Check sheet for the modelled part. Datum: model origin and axes. Units: mm. A direction names the side the tool comes from. Round coordinates to 2 decimals unless told otherwise and drop trailing zeros. Order: outer loops, then holes, each group sorted by start corner. A loop starts at its lowest first (then second) coordinate and runs counter-clockwise, first axis right, second up. Notation, with made-up numbers: (76, 30) -> (100, 30) arc R23 ccw to (100, 49) -> close; hole circle Ø7 at (56.25, -12.5). An arc over 180 degrees is marked (long way). Answer in a Markdown table with one row per item.
from build123d import *

# Parameters (mm, degrees)
BOSS_EXTRUDE1_DEPTH   = 6.35
SKETCH2_W             = 82.55
SKETCH2_H             = 9.525
BOSS_EXTRUDE2_DEPTH   = 50.8
CHAMFER1_SIZE         = 9.525
F_8_CLEARANCE_HOLE1_D = 4.9149
CUT_EXTRUDE1_REACH    = 223.791
SKETCH5_R             = 6.35
F_8_CLEARANCE_HOLE2_D = 4.9149
CHAMFER2_SIZE         = 2.54


with BuildPart() as part:
    # Sketch1 → Boss-Extrude1 (new body)
    with BuildSketch(Plane.XY):
        Polygon((-151.095016336, -53.975), (-126.488766336, -53.975), (-126.488766336, -25.4), (-209.038766336, -25.4), (-209.038766336, -53.975), align=None)
    extrude(amount=BOSS_EXTRUDE1_DEPTH)

    # Sketch2 → Boss-Extrude2 (add)
    with BuildSketch(Plane.XY.offset(6.35)):
        with Locations((-167.763766336, -30.1625)):
            Rectangle(SKETCH2_W, SKETCH2_H)
    extrude(amount=BOSS_EXTRUDE2_DEPTH)

    # Chamfer1
    chamfer1_edges = [part.edges().sort_by_distance(p)[0] for p in [
        (-167.763766336, -34.925, 6.35),
        (-126.488766336, -53.975, 3.175),
        (-126.488766336, -30.1625, 57.15),
        (-209.038766336, -30.1625, 57.15),
        (-209.038766336, -53.975, 3.175),
    ]]
    chamfer(chamfer1_edges, length=CHAMFER1_SIZE - 0.0001)  # a hair under: the kernel refuses the full size

    # #8 Clearance Hole1 (through all)
    with Locations(Plane.XY.offset(57.15)):
        with Locations((-193.163766336, -44.45), (-142.363766336, -44.45)):
            Hole(F_8_CLEARANCE_HOLE1_D / 2)

    # Sketch5 → Cut-Extrude1 (cut, up to next)
    with BuildSketch(Plane.XY.offset(6.35), mode=Mode.PRIVATE) as cut_extrude1_sk1:
        with Locations((-193.163766336, -44.45)):
            Circle(SKETCH5_R)
    cut_extrude1_tool1 = extrude(cut_extrude1_sk1.sketch, amount=CUT_EXTRUDE1_REACH, mode=Mode.PRIVATE) & part.part
    # Sketch5 → Cut-Extrude1 (cut, up to next)
    with BuildSketch(Plane.XY.offset(6.35), mode=Mode.PRIVATE) as cut_extrude1_sk2:
        with Locations((-142.363766336, -44.45)):
            Circle(SKETCH5_R)
    cut_extrude1_tool2 = extrude(cut_extrude1_sk2.sketch, amount=CUT_EXTRUDE1_REACH, mode=Mode.PRIVATE) & part.part
    add(cut_extrude1_tool1.solids().sort_by_distance((-193.163766, -44.45, 6.35))[0], mode=Mode.SUBTRACT)
    add(cut_extrude1_tool2.solids().sort_by_distance((-142.363766, -44.45, 6.35))[0], mode=Mode.SUBTRACT)

    # #8 Clearance Hole2 (through all)
    with Locations(Plane(origin=(0, -34.925, 0), x_dir=(-1, 0, 0), z_dir=(0, -1, 0))):
        with Locations((196.338766336, -41.818328597), (139.188766336, -41.818328597)):
            Hole(F_8_CLEARANCE_HOLE2_D / 2)

    # Chamfer2
    chamfer2_edges = [part.edges().sort_by_distance(p)[0] for p in [
        (-126.488766336, -34.92505, 0),
        (-167.763766336, -53.975, 0),
        (-204.276316336, -49.21255, 0),
        (-131.251216336, -49.21255, 0),
        (-209.038766336, -34.92505, 0),
        (-167.763766336, -25.4, 0),
    ]]
    chamfer(chamfer2_edges, length=CHAMFER2_SIZE)


solid = part.part
Item 1: Cross-section at B-B (y = -29.5). Record the boundary of the cut face in (x, z), and give its area (3 significant figures).
Result sheet:
| item | result |
|---|---|
| outline | (-209.04, 2.54) -> (-206.5, 0) -> (-129.03, 0) -> (-126.49, 2.54) -> (-126.49, 47.63) -> (-136.01, 57.15) -> (-199.51, 57.15) -> (-209.04, 47.63) -> close; hole circle Ø4.91 at (-196.34, 41.82); hole circle Ø4.91 at (-139.19, 41.82) |
| area | 4,580 mm^2 |
Item 2: Depth check by flat-ended pin: P1, Ø5.5, axis at x = -193.16, y = -44.45, coming from the +Z side; P2, Ø12.5, axis at x = -178, z = 46.5, coming from the -Y side (3 decimals); P3, Ø5, axis at x = -181, y = -43, coming from the +Z side. Enter the tip coordinate at first touch or a pass-through.
Result sheet:
| item | result |
|---|---|
| P1 | stops at z = 6.35 |
| P2 | stops at y = -34.925 |
| P3 | stops at z = 10.3 |
Item 3: Mould release check, pull along Z, two halves, no side actions. Record for faces 1 (the cylindrical face through (-136.845, -30.096, 41.08)), 2 (the flat face through (-209.039, -31, 20)), 3 (the cylindrical face through (-193.995, -30.096, 41.08)), 4 (the flat face through (-131.318, -30.229, 52.454)): pulls with the +Z half, pulls with the -Z half, needs draft (parallel to the pull), parting line crosses it, or undercut.
Result sheet:
| item | result |
|---|---|
| face 1 | undercut |
| face 2 | needs draft |
| face 3 | undercut |
| face 4 | pulls with the +Z half |
Item 4: Cross-section at C-C (x = -171). Record the boundary of the cut face in (y, z) (3 decimals).
Result sheet:
| item | result |
|---|---|
| outline | (-53.975, 2.54) -> (-51.435, 0) -> (-27.94, 0) -> (-25.4, 2.54) -> (-25.4, 57.15) -> (-34.925, 57.15) -> (-34.925, 15.875) -> (-44.45, 6.35) -> (-53.975, 6.35) -> close |
Item 5: Cross-section at A-A (z = 5). Record the boundary of the cut face in (x, y) (3 decimals).
Result sheet:
| item | result |
|---|---|
| outline | (-209.039, -44.45) -> (-199.514, -53.975) -> (-136.014, -53.975) -> (-126.489, -44.45) -> (-126.489, -25.4) -> (-209.039, -25.4) -> close; hole circle Ø4.915 at (-193.164, -44.45); hole circle Ø4.915 at (-142.364, -44.45) |
Item 6: Set-up check for faces 5 (the flat face through (-168, -48, 6.35)), 6 (the flat face through (-168.208, -52.723, 1.288)): record each of +Z, -Z, +X, -X, +Y, -Y from which the full face is reachable in a straight line by a thin tool's end or side.
Result sheet:
| item | result |
|---|---|
| face 5 | +Z, -Y |
| face 6 | -Z, +X, -X, -Y |
Item 7: Scan lines: line 1 (Z direction, x = -155, y = -46.25); line 2 (Y direction, x = -130.5, z = 38) (3 decimals). Record each from-to range of solid material in increasing order. Write a range as [from, to].
Result sheet:
| item | result |
|---|---|
| line 1 | z = [0, 6.35] |
| line 2 | y = [-34.925, -25.4] |
Item 8: Cross-section at D-D (y = -50.5). Record the boundary of the cut face in (x, z).
Result sheet:
| item | result |
|---|---|
| outline | (-202.99, 2.54) -> (-199.4, 0) -> (-136.13, 0) -> (-132.54, 2.54) -> (-132.54, 6.35) -> (-202.99, 6.35) -> close |
